Geometry check sheet. Reference: the model listing, model coordinates, mm. A direction names the side the tool comes from. Round coordinates to 2 decimals unless told otherwise and drop trailing zeros. Order: outer loops, then holes, each group sorted by start corner. A loop starts at its lowest first (then second) coordinate and runs counter-clockwise, first axis right, second up. Notation, with made-up numbers: (61.5, -19.5) -> (87.5, -19.5) arc R20 cw to (87.5, 15.5) -> close; hole circle Ø5 at (-6, 32). An arc over 180 degrees is marked (long way). Use a Markdown table: item, result. Add a question column.
Item 1: Material ranges on probe 1 along Y at (x, z) = (-17.5, 3.4); probe 2 along Y at (x, z) = (-17, 1); probe 3 along Z at (x, y) = (-15, 5.5), recorded low to high. Write a range as [from, to].
Item 2: Mould release check, pull along Y, two halves, no side actions. Record for faces 1 (the flat face through (-1, -30, 2)), 2 (the cylindrical face through (-16.47, -7.79, 2.46)), 3 (the cylindrical face through (-34.28, 24.93, 62)): pulls with the +Y half, pulls with the -Y half, needs draft (parallel to the pull), parting line crosses it, or undercut.
Item 3: Set-up check for faces 4 (the cylindrical face through (-16.2, 8.06, 2.46)), 5 (the flat face through (-18, 20, 21)), 6 (the flat face through (-24.44, 24.93, 51.49)): record each of +Z, -Z, +X, -X, +Y, -Y from which the full face is reachable in a straight line by a thin tool's end or side.
Item 4: Gauge pin test, flat ends, axial feed: pin 1 Ø14.5 at (x, y) = (0, 0) entering from +Z; pin 2 Ø4 at (x, z) = (1.89, 12.44) entering from -Y; pin 3 Ø4 at (x, y) = (17.5, -7) entering from +Z. Record the tip position at first contact, or that the pin passes through.
Item 5: Sectioned sample at A-A, the plane y = 0. Record the cut outline in (x, z).
Item 6: Sectioned sample at B-B, the plane z = 40. Record the cut outline in (x, y), and give its area (3 significant figures).
Item 7: Sectioned sample at D-D, the plane y = -7. Record the cut outline in (x, z), and give its area (3 significant figures).
Item 8: Sectioned sample at C-C, the plane x = 26. Record the cut outline in (y, z), and give its area (4 significant figures).
from build123d import *

# Parameters (mm, degrees)
SZKIC1_W                    = 80
SZKIC1_H                    = 60
DODANIE_WYCI_GNI_CIE1_DEPTH = 5
DODANIE_WYCI_GNI_CIE2_DEPTH = 10
OTW_R_POD_RUB_M22_D         = 2.6
OTW_R_POD_RUB_M22_DEPTH     = 5
WYTNIJ_WYCI_GNI_CIE2_REACH  = 12
OTW_R_POD_RUB_M21_D         = 2.6
OTW_R_POD_RUB_M21_DEPTH     = 10
ZAOKR_GLENIE5_R             = 10
OTW_R_POD_RUB_M201_D        = 24
OTW_R_POD_RUB_M201_DEPTH    = 5


with BuildPart() as part:
    # Szkic1 → Dodanie-wyciągnięcie1 (new body)
    with BuildSketch(Plane.XY):
        Rectangle(SZKIC1_W, SZKIC1_H)
    extrude(amount=DODANIE_WYCI_GNI_CIE1_DEPTH)

    # Szkic2 → Dodanie-wyciągnięcie2 (add)
    with BuildSketch(Plane(origin=(0, 30, 0), x_dir=(1, 0, 0), z_dir=(0, 1, 0))):
        Polygon((40, 0), (-40, 0), (-40, -75), (40, -5), align=None)
    extrude(amount=-DODANIE_WYCI_GNI_CIE2_DEPTH)

    # Otwór pod śrubę M22
    with Locations(Plane(origin=(-17.5, 8, 5), x_dir=(1, 0, 0), z_dir=(0, 0, 1))):
        with Locations((0, 0), (0, -15), (35, 0), (35, -15)):
            Hole(OTW_R_POD_RUB_M22_D / 2, depth=OTW_R_POD_RUB_M22_DEPTH)

    # Szkic17 → Wytnij-wyciągnięcie2 (cut, up to next)
    with BuildSketch(Plane.XZ.offset(-20), mode=Mode.PRIVATE) as wytnij_wyci_gni_cie2_sk1:
        Polygon((-36, 38.280794335), (-5.144355517, 11.282105413), (8.684241248, 27.086216001), (-22.171403235, 54.084904924), (-26.78093549, 48.816868061), (-29.414953921, 51.121634189), (-34.024486176, 45.853597326), (-31.390467745, 43.548831198), align=None)
    wytnij_wyci_gni_cie2_tool1 = extrude(wytnij_wyci_gni_cie2_sk1.sketch, amount=-WYTNIJ_WYCI_GNI_CIE2_REACH, mode=Mode.PRIVATE) & part.part
    add(wytnij_wyci_gni_cie2_tool1.solids().sort_by_distance((-14.121175, 20, 33.088889))[0], mode=Mode.SUBTRACT)

    # Otwór pod śrubę M21
    with Locations(Plane(origin=(0, 20, 0), x_dir=(-1, 0, 0), z_dir=(0, -1, 0))):
        with Locations((35.576675609, -45.21861074), (28.991629531, -52.744377687), (-8.471638332, -19.964018307), (-1.886592253, -12.43825136)):
            Hole(OTW_R_POD_RUB_M21_D / 2, depth=OTW_R_POD_RUB_M21_DEPTH)

    # Zaokrąglenie5
    zaokr_glenie5_edges = [part.edges().sort_by_distance(p)[0] for p in [
        (-40, 25, 75),
    ]]
    fillet(zaokr_glenie5_edges, radius=ZAOKR_GLENIE5_R)

    # Otwór pod śrubę M201
    with Locations(Plane(origin=(0, 0, 0), x_dir=(-1, 0, 0), z_dir=(0, 0, -1))):
        with Locations((0, 0)):
            Hole(OTW_R_POD_RUB_M201_D / 2, depth=OTW_R_POD_RUB_M201_DEPTH)


solid = part.part
Found:
| question | item | result |
|---|---|---|
| 1 | probe 1 | y = [-30, -8.3], [-5.7, 6.7], [9.3, 30] |
| 1 | probe 2 | y = [-30, -8.2], [-5.8, 6.8], [9.2, 30] |
| 1 | probe 3 | z = [0, 5] |
| 2 | face 1 | pulls with the -Y half |
| 2 | face 2 | undercut |
| 2 | face 3 | needs draft |
| 3 | face 4 | +Z, -Z |
| 3 | face 5 | +Z, +X, -X, -Y |
| 3 | face 6 | +Y, -Y |
| 4 | pin 1 | passes through |
| 4 | pin 2 | stops at y = 20 |
| 4 | pin 3 | stops at z = 5 |
| 5 | outline | (-40, 0) -> (-12, 0) -> (-12, 5) -> (-40, 5) -> close; (12, 0) -> (40, 0) -> (40, 5) -> (12, 5) -> close |
| 6 | outline | (-40, 20) -> (-34.5, 20) -> (-34.5, 30) -> (-40, 30) -> close; (-6.07, 20) -> (0, 20) -> (0, 30) -> (-6.07, 30) -> close |
| 6 | area | 116 mm2 |
| 7 | outline | (-40, 0) -> (-18.8, 0) -> (-18.8, 5) -> (-40, 5) -> close; (-16.2, 0) -> (-9.75, 0) -> (-9.75, 5) -> (-16.2, 5) -> close; (9.75, 0) -> (16.2, 0) -> (16.2, 5) -> (9.75, 5) -> close; (18.8, 0) -> (40, 0) -> (40, 5) -> (18.8, 5) -> close |
| 7 | area | 277 mm2 |
| 8 | outline | (-30, 0) -> (30, 0) -> (30, 17.25) -> (20, 17.25) -> (20, 5) -> (-30, 5) -> close |
| 8 | area | 422.5 mm2 |
